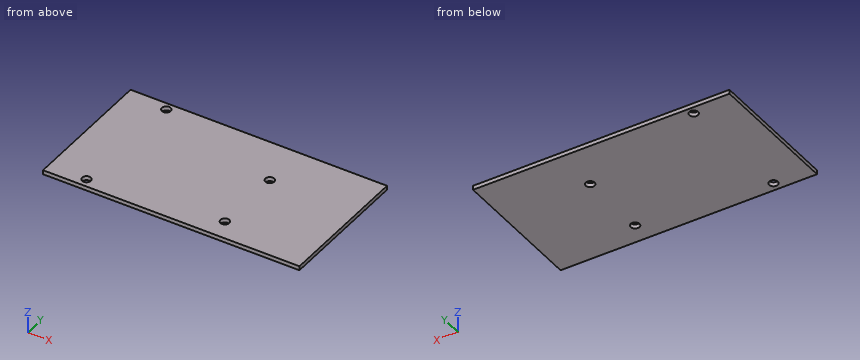
Solid Edge part; units mm, degrees
sketch "Sketch1" plane through (0, 0, 0) normal (0, 0, 1) x (1, 0, 0)
  line L0 (-50.8, -27.178) -> (50.8, -27.178)
  line L1 (50.8, -27.178) -> (50.8, 27.178)
  line L2 (50.8, 27.178) -> (-50.8, 27.178)
  line L3 (-50.8, 27.178) -> (-50.8, -27.178)
extrude "Protrusion1" add sketch "Sketch1" against normal blind 1.65
sketch "Sketch2" plane through (0, 0, 0) normal (0, 0, 1) x (1, 0, 0)
  circle A0 centre (-34.69, 24.132) radius 1.75
  circle A1 centre (-35.8, -23.678) radius 1.75
  circle A2 centre (16.09, -19.058) radius 1.75
  circle A3 centre (16.09, 8.842) radius 1.75
extrude "Cutout1" cut sketch "Sketch2" against normal up to vertex (1.65 mm away)
Geometry: final body of the model. Coordinates: model frame, mm. Round coordinates to 2 decimals unless told otherwise and drop trailing zeros. Order: outer loops, then holes, each group sorted by start corner. A loop starts at its lowest first (then second) coordinate and runs counter-clockwise, first axis right, second up. Notation, with made-up numbers: (20, -30) -> (38, -30) arc R19 cw to (38, -15) -> close; hole circle Ø6 at (82.25, -17.5). An arc over 180 degrees is marked (long way). Use CSV: the item, a comma, the result in double quotes. Start each with the question number.
1) First-contact query: pin 1 Ø3 at (x, y) = (16.09, 8.842) entering from +Z. Flat tip, straight axial feed; report the tip coordinate or a pass-through.
2) Material intervals for line 1 along Y through (x, z) = (-35.8, -1.1); line 2 along X through (y, z) = (8.5, -0.1); line 3 along X through (y, z) = (-23, -0.9), sorted ascending. Write a range as from..to.
3) Section A-A (x = 16.09). Return the cut outline in (y, z).
Returned:
1,pin 1,"passes through"
2,line 1,"y = -27.18..-25.43, -21.93..22.78, 25.48..27.18"
2,line 2,"x = -50.8..14.37, 17.81..50.8"
2,line 3,"x = -50.8..-37.41, -34.19..50.8"
3,outline,"(-27.18, -1.65) -> (-20.81, -1.65) -> (-20.81, 0) -> (-27.18, 0) -> close; (-17.31, -1.65) -> (7.09, -1.65) -> (7.09, 0) -> (-17.31, 0) -> close; (10.59, -1.65) -> (27.18, -1.65) -> (27.18, 0) -> (10.59, 0) -> close"
